Work out the finished part from the listing and answer in its coordinate system (mm). Coordinates: 2 decimals unless noted, no trailing zeros. Order: outer loops, then holes, each group sorted by start corner. A loop starts at its lowest first (then second) coordinate and runs counter-clockwise, first axis right, second up. Notation, with made-up numbers: M 44,65 L 88,65 A21 cw 88,91 Z; hole C 9,-30.75 d1. An arc over 180 degrees is marked long. Answer in a Markdown table with one row per item. Add a question column.
Item 1: The part is cut by section A-A (z = 4.5). Write down the section's boundary in (x, y).
Item 2: A flat-ended cylindrical pin translates along its axis: pin 1 Ø3.5 at (x, z) = (27, 9) entering from +Y. Find the tip coordinate at first contact, or state that the pin passes through.
Item 3: Consider line 1 (Y direction, x = 27.5, z = 7); line 2 (Y direction, x = -18.5, z = 10.75); line 3 (X direction, y = 55, z = 16.25). Determine where each line is inside the solid, lowest interval first. Write a range as from..to.
from build123d import *

# Parameters (mm, degrees)
F1_DEPTH = 25.4


with BuildPart() as f1:
    # F0 (on Top) → F1 (new body)
    with BuildSketch(Plane.XY):
        with BuildLine():
            ThreePointArc((24.54447, 55.661607), (24.536622, 55.977219), (24.513096, 56.292051))
            Line((24.513096, 56.292051), (-24.513096, 56.292051))
            ThreePointArc((-24.513096, 56.292051), (-24.536622, 55.977219), (-24.54447, 55.661607))
            Line((-24.54447, 55.661607), (-24.54447, 50.572495))
            Line((-24.54447, 50.572495), (24.54447, 50.572495))
            Line((24.54447, 50.572495), (24.54447, 55.661607))
        make_face()
        with BuildLine():
            ThreePointArc((35.280632, 49.942051), (33.42076, 54.432179), (28.930632, 56.292051))
            Line((28.930632, 56.292051), (24.513096, 56.292051))
            ThreePointArc((24.513096, 56.292051), (24.536622, 55.977219), (24.54447, 55.661607))
            Line((24.54447, 55.661607), (24.54447, 50.572495))
            Line((24.54447, 50.572495), (-24.54447, 50.572495))
            Line((-24.54447, 50.572495), (-24.54447, 55.661607))
            ThreePointArc((-24.54447, 55.661607), (-24.536622, 55.977219), (-24.513096, 56.292051))
            Line((-24.513096, 56.292051), (-28.930632, 56.292051))
            ThreePointArc((-28.930632, 56.292051), (-33.42076, 54.432179), (-35.280632, 49.942051))
            Line((-35.280632, 49.942051), (-35.280632, -49.942051))
            ThreePointArc((-35.280632, -49.942051), (-33.42076, -54.432179), (-28.930632, -56.292051))
            Line((-28.930632, -56.292051), (28.930632, -56.292051))
            ThreePointArc((28.930632, -56.292051), (33.42076, -54.432179), (35.280632, -49.942051))
            Line((35.280632, -49.942051), (35.280632, 49.942051))
        make_face()
        with BuildLine():
            Line((-24.513096, 56.292051), (24.513096, 56.292051))
            ThreePointArc((24.513096, 56.292051), (22.455877, 60.369357), (18.19447, 62.011607))
            Line((18.19447, 62.011607), (-18.19447, 62.011607))
            ThreePointArc((-18.19447, 62.011607), (-22.455877, 60.369357), (-24.513096, 56.292051))
        make_face()
    extrude(amount=F1_DEPTH)


solid = f1.part
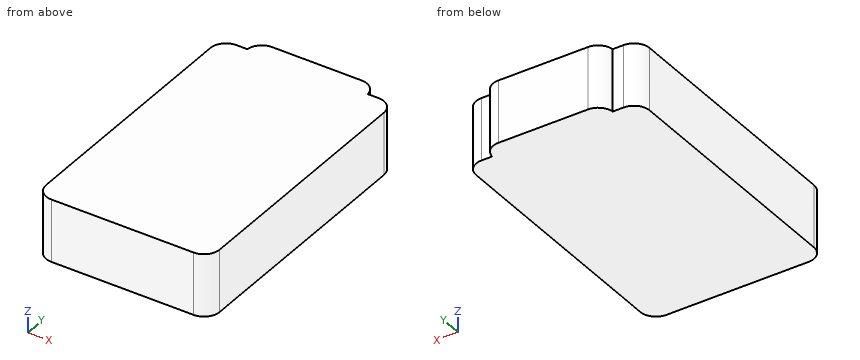
Reply:
| question | item | result |
|---|---|---|
| 1 | outline | M -35.28,-49.94 A6.35 ccw -28.93,-56.29 L 28.93,-56.29 A6.35 ccw 35.28,-49.94 L 35.28,49.94 A6.35 ccw 28.93,56.29 L 24.51,56.29 A6.35 ccw 18.19,62.01 L -18.19,62.01 A6.35 ccw -24.51,56.29 L -28.93,56.29 A6.35 ccw -35.28,49.94 Z |
| 2 | pin 1 | stops at y = 56.29 |
| 3 | line 1 | y = -56.29..56.29 |
| 3 | line 2 | y = -56.29..62 |
| 3 | line 3 | x = -32.77..32.77 |
